from build123d import *

# Parameters (mm, degrees)
F0_W     = 44.7
F0_H     = 40.1
F0_R     = 5
F0_R_2   = 8.3
F1_DEPTH = 8
F2_DEPTH = 4
F0_R_3   = 4
F3_DEPTH = 1
F4_R     = 1.99999


# Not quite as in the source:
# - a fillet or chamfer is up to 0.001 mm smaller than in the source, because OpenCascade refuses the exact size


with BuildPart() as f1:
    # F0 (on Top) → F1 (new body)
    with BuildSketch(Plane.XY):
        Rectangle(F0_W, F0_H)
        with Locations((-15.35, -12.05)):
            Circle(F0_R, mode=Mode.SUBTRACT)
        with Locations((15.35, -12.05)):
            Circle(F0_R, mode=Mode.SUBTRACT)
        Circle(F0_R_2, mode=Mode.SUBTRACT)
        with Locations((-15.35, 12.05)):
            Circle(F0_R, mode=Mode.SUBTRACT)
        with Locations((15.35, 12.05)):
            Circle(F0_R, mode=Mode.SUBTRACT)
    extrude(amount=F1_DEPTH)

    # F0 (on Top) → F2 (join)
    with BuildSketch(Plane.XY):
        Circle(F0_R_2)
    extrude(amount=F2_DEPTH)

    # F0 (on Top) → F3 (join)
    with BuildSketch(Plane.XY):
        with Locations((15.35, 12.05)):
            Circle(F0_R)
        with Locations((15.35, 12.05)):
            Circle(F0_R_3, mode=Mode.SUBTRACT)
        with Locations((15.35, -12.05)):
            Circle(F0_R)
        with Locations((15.35, -12.05)):
            Circle(F0_R_3, mode=Mode.SUBTRACT)
        with Locations((-15.35, -12.05)):
            Circle(F0_R)
        with Locations((-15.35, -12.05)):
            Circle(F0_R_3, mode=Mode.SUBTRACT)
        with Locations((-15.35, 12.05)):
            Circle(F0_R)
        with Locations((-15.35, 12.05)):
            Circle(F0_R_3, mode=Mode.SUBTRACT)
    extrude(amount=F3_DEPTH)

    # F4 (radius 2 in the source; OpenCascade refuses exactly that, so slightly less here)
    f4_edges = [f1.edges().sort_by_distance(p)[0] for p in [
        (0, 20.05, 8),
        (-22.35, 0, 8),
        (0, -20.05, 8),
        (22.35, 0, 8),
        (0, -20.05, 0),
        (-22.35, 0, 0),
        (-22.35, -20.05, 4),
        (22.35, -20.05, 4),
        (22.35, 0, 0),
        (22.35, 20.05, 4),
        (0, 20.05, 0),
        (-22.35, 20.05, 4),
    ]]
    fillet(f4_edges, radius=F4_R)


solid = f1.part
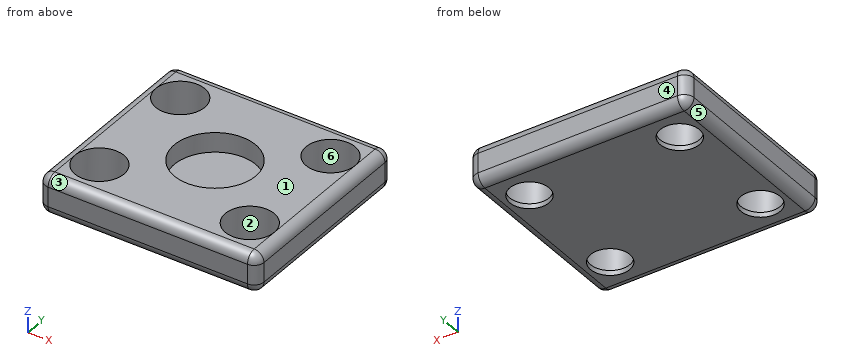
For this review, take the finished solid that the model builds, in its own axes (mm). Face numbers are marked on the shaded views. A direction names the side the tool comes from. Round coordinates to 2 decimals unless told otherwise and drop trailing zeros. Write each loop counter-clockwise with the first axis right and the second up, starting at its lowest first coordinate (ties: lowest second). Pieces come first, ordered by that corner, then holes. Notation, with made-up numbers: (53.5, 62.25) - (69.5, 62.25) arc R6 ccw to (69.5, 73.25) - close; hole circle Ø7 at (32.25, 53.25). An arc over 180 degrees is marked (long way). Write item = value, one per line. Start each with the question number.
1. Wall thickness on L1, parallel to Y at x = 15.35, z = 6; L2, parallel to X at y = 14, z = 5.75; L3, parallel to Y at x = 15.35, z = 0.6: over which ranges is each line inside the solid? List them lowest first.
2. For pin 1 Ø5 at (x, y) = (16.5, 14) entering from +Z, flat-tipped, find the tip position at first contact; note if it passes through.
3. Consider section C-C on z = 4.5. State the section outline as (x, y) points, plus the area to 3 significant figures.
4. Consider section B-B on y = -12.05. Give the number of separate pieces and of enclosed holes in the cut face, plus the area to 3 significant figures.
5. Consider section D-D on y = 0. State the section outline as (x, z) points.
6. Draft analysis for pull direction Y (two halves, no side actions). For the marked faces 1, 2, 3 and 4, state which applies: released by +Y, released by -Y, zero draft, split by the parting line, or undercut.
7. Consider section A-A on x = 15.35. State the section outline as (y, z) points.
8. For the marked faces 5 and 6, list the 3-axis set-ups (+Z, -Z, +X, -X, +Y, -Y) from which the entire face can be reached by the end or side of a thin tool; tool diameter is ignored.
Evaluation:
q1.L1 = -20.05 to -17.05, -7.05 to 7.05, 17.05 to 20.05
q1.L2 = -22.35 to -19.95, -10.75 to 10.75, 19.95 to 22.35
q1.L3 = -19.48 to -16.05, -8.05 to 8.05, 16.05 to 19.48
q2.pin_1 = 1
q3.outline = (-22.35, -18.05) arc R2 ccw to (-20.35, -20.05) - (20.35, -20.05) arc R2 ccw to (22.35, -18.05) - (22.35, 18.05) arc R2 ccw to (20.35, 20.05) - (-20.35, 20.05) arc R2 ccw to (-22.35, 18.05) - close; hole circle Ø10 at (-15.35, -12.05); hole circle Ø10 at (-15.35, 12.05); hole circle Ø16.6 at (0, 0); hole circle Ø10 at (15.35, -12.05); hole circle Ø10 at (15.35, 12.05)
q3.area = 1,260 mm2
q4.separate_pieces = 3
q4.enclosed_holes = 0
q4.area = 198 mm2
q5.outline = (-22.35, 2) arc R2 ccw to (-20.35, 0) - (20.35, 0) arc R2 ccw to (22.35, 2) - (22.35, 6) arc R2 ccw to (20.35, 8) - (8.3, 8) - (8.3, 4) - (-8.3, 4) - (-8.3, 8) - (-20.35, 8) arc R2 ccw to (-22.35, 6) - close
q6.face_1 = zero draft
q6.face_2 = undercut
q6.face_3 = released by -Y
q6.face_4 = released by +Y
q7.outline = (-20.05, 2) arc R2 ccw to (-18.05, 0) - (-16.05, 0) - (-16.05, 1) - (-17.05, 1) - (-17.05, 8) - (-18.05, 8) arc R2 ccw to (-20.05, 6) - close; (-8.05, 0) - (8.05, 0) - (8.05, 1) - (7.05, 1) - (7.05, 8) - (-7.05, 8) - (-7.05, 1) - (-8.05, 1) - close; (16.05, 0) - (18.05, 0) arc R2 ccw to (20.05, 2) - (20.05, 6) arc R2 ccw to (18.05, 8) - (17.05, 8) - (17.05, 1) - (16.05, 1) - close
q8.face_5 = -Z, -X, +Y, -Y
q8.face_6 = +Z
